For this review, take the finished solid that the model builds, in its own axes (mm). Face numbers are marked on the shaded views. A direction names the side the tool comes from. Coordinates: 2 decimals unless noted, no trailing zeros. Loops run counter-clockwise (first coordinate to the right, second up) from the corner with the lowest first, then second, coordinate; pieces in that order, holes last. Notation, with made-up numbers: (66, 36) - (85, 36) arc R33 ccw to (85, 68) - close; hole circle Ø9 at (62, 30.25). An arc over 180 degrees is marked (long way). One line per item, written item: value. Start each with the question number.
1. Take a section at A-A, the plane z = 5. State the section outline as (x, y) points.
2. To check wall thickness, follow line 1 (Y direction, x = 18.75, z = -9.5); line 2 (X direction, y = 8.5, z = -17); line 3 (Z direction, x = 5.5, y = -0.5). State the ranges of each line that lie inside material, in increasing order. Write a range as from..to.
3. Insertion check: pin 1 (1.5 mm diameter, centred on x = 15, z = -10, fed in from -Y); pin 2 (3 mm diameter, centred on x = 17.5, z = -10, fed in from +Y); pin 3 (1 mm diameter, centred on x = 4, z = 7, fed in from +Y); pin 4 (8 mm diameter, centred on x = 15.5, y = -0.5, fed in from -Z). Each pin has a flat end and moves straight along its axis. Give the tip position at first contact, or say it passes through.
4. Take a section at D-D, the plane y = -12.5. State the section outline as (x, z) points.
5. For the marked faces 1, 2 and 3, list the 3-axis set-ups (+Z, -Z, +X, -X, +Y, -Y) from which the entire face can be reached by the end or side of a thin tool; tool diameter is ignored.
6. Take a section at C-C, the plane z = 0. State the section outline as (x, y) points, and give its area (3 significant figures).
7. Take a section at B-B, the plane x = 13.25. State the section outline as (y, z) points.
```python
from build123d import *

# Parameters (mm, degrees)
SKETCH2_R           = 20
BOSS_EXTRUDE1_DEPTH = 10
BOSS_EXTRUDE2_DEPTH = 10


with BuildPart() as part:
    # Sketch2 → Boss-Extrude1 (new body)
    with BuildSketch(Plane(origin=(0, 0, 0), x_dir=(0, 0, -1), z_dir=(1, 0, 0))):
        Circle(SKETCH2_R)
    extrude(amount=BOSS_EXTRUDE1_DEPTH)

    # Sketch3 → Boss-Extrude2 (add)
    with BuildSketch(Plane(origin=(10, 0, 0), x_dir=(0, 0, -1), z_dir=(1, 0, 0))):
        with BuildLine():
            Line((19.364916731, 5), (-19.364916731, 5))
            ThreePointArc((-19.364916731, 5), (-20, 0), (-19.364916731, -5))
            Line((-19.364916731, -5), (19.364916731, -5))
            ThreePointArc((19.364916731, -5), (20, 0), (19.364916731, 5))
        make_face()
    extrude(amount=BOSS_EXTRUDE2_DEPTH)


solid = part.part
```
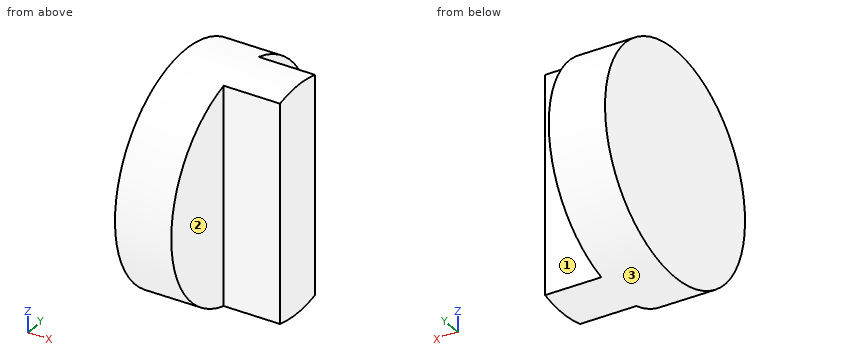
Solutions:
1. outline: (0, -19.36) - (10, -19.36) - (10, -5) - (20, -5) - (20, 5) - (10, 5) - (10, 19.36) - (0, 19.36) - close
2. line 1: -5..5
2. line 2: 0..10
2. line 3: -19.99..19.99
3. pin 1: y = -5
3. pin 2: y = 5
3. pin 3: y = 18.91
3. pin 4: z = -20
4. outline: (0, -15.61) - (10, -15.61) - (10, 15.61) - (0, 15.61) - close
5. face 1: +Z, -Z, +X, +Y
5. face 2: +Z, -Z, +X, -Y
5. face 3: +X, -X
6. outline: (0, -20) - (10, -20) - (10, -5) - (20, -5) - (20, 5) - (10, 5) - (10, 20) - (0, 20) - close
6. area: 500 mm2
7. outline: (-5, -19.36) arc R20 ccw to (5, -19.36) - (5, 19.36) arc R20 ccw to (-5, 19.36) - close
